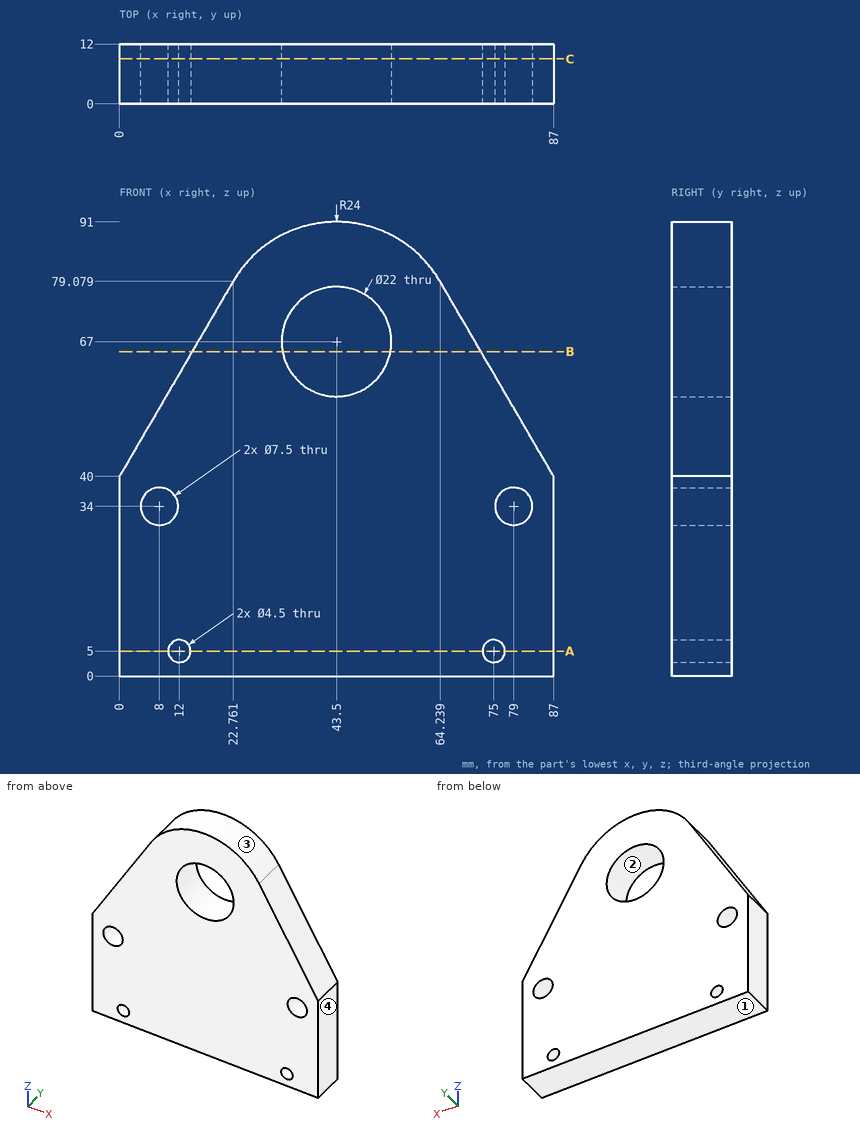
Study the drawing (mm; zero at the part's minimum x, y, z) and answer. Give positions to 0.01 mm unless a question says otherwise; leave off trailing zeros. Order: outer loops, then holes, each group sorted by start corner. A loop starts at its lowest first (then second) coordinate and runs counter-clockwise, first axis right, second up. Notation, with made-up numbers: (80, -25.75) - (126, -25.75) arc R37 ccw to (126, 12.25) - close; hole circle Ø6 at (23.5, 32.5). An arc over 180 degrees is marked (long way). Answer as CSV lines item,"result". Start each with the question number.
Q1. The mould has two halves that part along X. Classify the marked faces 1, 2, 3 and 4: +X half, -X half, draft (parallel to the pull), parting line (faces both ways), or undercut.
Q2. The part is cut by section C-C (y = 9). Write down the section's boundary in (x, z), then the cut area to 3 significant figures.
Q3. Given pin 1 Ø1 at (y, z) = (1.5, 61.5) entering from -X, flat-ended and moving along its own axis, determine where the tip first touches the part or whether it passes through.
Q4. The part is cut by section A-A (z = 5). Write down the section's boundary in (x, y).
Q5. The part is cut by section B-B (z = 65). Write down the section's boundary in (x, y).
Q6. Find the intervals of material crossed by L1, parallel to X at y = 4.75, z = 6.5; L2, parallel to Z at x = 10, y = 11.5; L3, parallel to X at y = 4.25, z = 76 (1 decimal), in increasing order. Write a range as [from, to].
Check result:
1,face 1,"draft"
1,face 2,"undercut"
1,face 3,"parting line"
1,face 4,"+X half"
2,outline,"(0, 0) - (87, 0) - (87, 40) - (64.24, 79.08) arc R24 ccw to (22.76, 79.08) - (0, 40) - close; hole circle Ø7.5 at (8, 34); hole circle Ø4.5 at (12, 5); hole circle Ø22 at (43.5, 67); hole circle Ø4.5 at (75, 5); hole circle Ø7.5 at (79, 34)"
2,area,"5,840 mm²"
3,pin 1,"stops at x = 12.23"
4,outline,"(0, 0) - (9.75, 0) - (9.75, 12) - (0, 12) - close; (14.25, 0) - (72.75, 0) - (72.75, 12) - (14.25, 12) - close; (77.25, 0) - (87, 0) - (87, 12) - (77.25, 12) - close"
5,outline,"(14.56, 0) - (32.68, 0) - (32.68, 12) - (14.56, 12) - close; (54.32, 0) - (72.44, 0) - (72.44, 12) - (54.32, 12) - close"
6,L1,"x = [0, 10.32], [13.68, 73.32], [76.68, 87]"
6,L2,"z = [0, 3.97], [6.03, 30.83], [37.17, 57.17]"
6,L3,"x = [21, 37.2], [49.8, 66]"
